Read the model definition and answer for the solid it produces. Units are mm, in the model's axes. Face numbers are marked on the shaded views. A direction names the side the tool comes from. Coordinates: 2 decimals unless noted, no trailing zeros. Order: outer loops, then holes, each group sorted by start corner. A loop starts at its lowest first (then second) coordinate and runs counter-clockwise, first axis right, second up. Notation, with made-up numbers: (79, -6.75) - (120, -6.75) arc R11 cw to (120, 9.25) - close; hole circle Ø11 at (56.5, -35). An arc over 180 degrees is marked (long way). Use one line per item in the form item = value.
```python
from build123d import *

# Parameters (mm, degrees)
EXTRUDE_THIN1_DEPTH = 20
FILLET1_R           = 3
SKETCH2_R           = 1.5
CUT_EXTRUDE1_DEPTH  = 270


with BuildPart() as part:
    # Sketch1 → Extrude-Thin1 (new body)
    with BuildSketch(Plane(origin=(0, 0, 0), x_dir=(1, 0, 0), z_dir=(0, 1, 0))):
        Polygon((0, 80), (0, 0), (225, 0), (225, 80), (227.5, 80), (227.5, -2.5), (-2.5, -2.5), (-2.5, 80), align=None)
    extrude(amount=EXTRUDE_THIN1_DEPTH)

    # Fillet1
    fillet1_edges = [part.edges().sort_by_distance(p)[0] for p in [
        (227.5, 10, 2.5),
        (-2.5, 10, 2.5),
        (0, 10, 0),
        (225, 10, 0),
    ]]
    fillet(fillet1_edges, radius=FILLET1_R)

    # Sketch2 → Cut-Extrude1 (cut)
    with BuildSketch(Plane(origin=(-2.5, 0, 0), x_dir=(0, 0, -1), z_dir=(1, 0, 0))):
        with Locations((70, 15)):
            Circle(SKETCH2_R)
        with Locations((70, 5)):
            Circle(SKETCH2_R)
    extrude(amount=CUT_EXTRUDE1_DEPTH, mode=Mode.SUBTRACT)


solid = part.part
```
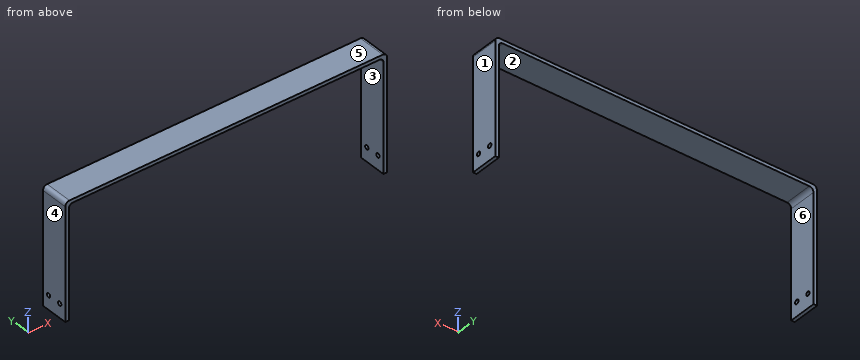
(1) Given pin 1 Ø1 at (x, y) = (61.5, 14.5) entering from -Z; pin 2 Ø3.5 at (y, z) = (5, -70) entering from +X; pin 3 Ø1.8 at (y, z) = (15, -70) entering from +X, each flat-ended and moving along its own axis, determine where each tip first touches the part or whether it passes through.
Answer list:
pin_1 = 0
pin_2 = 227.5
pin_3 = through
(2) The mould has two halves that part along X. Classify the marked faces 1, 2, 3 and 4: +X half, -X half, draft (parallel to the pull), parting line (faces both ways), or undercut.
Answer list:
face_1 = +X half
face_2 = undercut
face_3 = undercut
face_4 = -X half
(3) Straight lines are drawn through the part: L1, parallel to Y at x = -1, z = -70; L2, parallel to X at y = 9.5, z = -44.5; L3, parallel to Z at x = 110, y = 11.5. For each, find the intervals that lie inside material, in ascending order.
Answer list:
L1 = 0 to 3.5, 6.5 to 13.5, 16.5 to 20
L2 = -2.5 to 0, 225 to 227.5
L3 = 0 to 2.5
(4) Section C-C, the plane x = 119 is taken. Write down the section's boundary in (y, z), then the cut area to 3 significant figures.
Answer list:
outline = (0, 0) - (20, 0) - (20, 2.5) - (0, 2.5) - close
area = 50.0 mm2
(5) Section A-A, the plane z = -42.5 is taken. Write down the section's boundary in (x, y), then the cut area to 3 significant figures.
Answer list:
outline = (-2.5, 0) - (0, 0) - (0, 20) - (-2.5, 20) - close; (225, 0) - (227.5, 0) - (227.5, 20) - (225, 20) - close
area = 100 mm2
(6) Which of the six approach directions +Z, -Z, +X, -X, +Y, -Y give full straight-line access (tool end or side, diameter ignored) to the marked faces 5 and 6?
Answer list:
face_5 = +Z, +X, -X, +Y, -Y
face_6 = -Z, +Y, -Y
(7) Section B-B, the plane y = 9 is taken. Write down the section's boundary in (x, z), then the cut area to 3 significant figures.
Answer list:
outline = (-2.5, -80) - (0, -80) - (0, -3) arc R3 cw to (3, 0) - (222, 0) arc R3 cw to (225, -3) - (225, -80) - (227.5, -80) - (227.5, -0.5) arc R3 ccw to (224.5, 2.5) - (0.5, 2.5) arc R3 ccw to (-2.5, -0.5) - close
area = 975 mm2
